Read the model definition and answer for the solid it produces. Units are mm, in the model's axes. Coordinates: 2 decimals unless noted, no trailing zeros. Order: outer loops, then holes, each group sorted by start corner. A loop starts at its lowest first (then second) coordinate and runs counter-clockwise, first axis right, second up. Notation, with made-up numbers: (46.5, 6.25) -> (52.5, 6.25) arc R28 cw to (52.5, 35.25) -> close; hole circle Ø7 at (35.25, -1.5). An arc over 180 degrees is marked (long way). Return JSON: item names as keys, results as strings. Group by question number.
```python
from build123d import *

# Parameters (mm, degrees)
F0_W     = 647.7
F0_H     = 88.9
F1_DEPTH = 19.05
F3_DEPTH = 127
F5_DEPTH = 127


with BuildPart() as f1:
    # F0 (on Front) → F1 (new body)
    with BuildSketch(Plane.XZ):
        with Locations((-323.85, 44.45)):
            Rectangle(F0_W, F0_H)
    extrude(amount=F1_DEPTH)

    # F2 (on face) → F3 (cut)
    with BuildSketch(Plane.XY.offset(88.9)):
        Polygon((-647.7, 0), (-647.7, -19.05), (-628.65, 0), align=None)
    extrude(amount=-F3_DEPTH, mode=Mode.SUBTRACT)

    # F4 (on face) → F5 (cut)
    with BuildSketch(Plane.XY.offset(88.9)):
        Polygon((-19.05, 0), (0, -19.05), (0, 0), align=None)
    extrude(amount=-F5_DEPTH, mode=Mode.SUBTRACT)


solid = f1.part
```
1. Find section B-B on z = 81. Determine the outline of the cut face in (x, y), and give its area (3 significant figures).
2. Find section A-A on y = -11. Determine the outline of the cut face in (x, z).
3. Given pin 1 (1 mm diameter, centred on y = -14, z = 22, fed in from -X); pin 2 (2 mm diameter, centred on y = -6.5, z = 67, fed in from +X); pin 3 (10 mm diameter, centred on y = -10, z = 26, fed in from +X), each flat-ended and moving along its own axis, determine where each tip first touches the part or whether it passes through.
4. Straight lines are drawn through the part: L1, parallel to X at y = -15.25, z = 51; L2, parallel to X at y = -14.25, z = 48.5. For each, find the intervals that lie inside material, in ascending order.
Result:
{
 "1": {"outline": "(-647.7, -19.05) -> (0, -19.05) -> (-19.05, 0) -> (-628.65, 0) -> close", "area": "12,000 mm^2"},
 "2": {"outline": "(-639.65, 0) -> (-8.05, 0) -> (-8.05, 88.9) -> (-639.65, 88.9) -> close"},
 "3": {"pin 1": "x = -643.15", "pin 2": "x = -11.55", "pin 3": "x = -4.05"},
 "4": {"L1": "-643.9 to -3.8", "L2": "-642.9 to -4.8"}
}
